Read the model definition and answer for the solid it produces. Units are mm, in the model's axes. A direction names the side the tool comes from. Coordinates: 2 decimals unless noted, no trailing zeros. Write each loop counter-clockwise with the first axis right and the second up, starting at its lowest first coordinate (ties: lowest second). Pieces come first, ordered by that corner, then holes. Notation, with made-up numbers: (-40, 67) -> (9, 67) arc R19 cw to (9, 82) -> close; hole circle Ø3 at (6.5, 74). An arc over 180 degrees is marked (long way). One line per item, written item: value. Start each with the question number.
1. For a pull along X with two mould halves and no side action, classify faces 3 (the flat face through (74, 18, 0)), 4 (the flat face through (23, 69, 337)), 5 (the cylindrical face through (90.178, 81.787, 127.677)) as pulls with the +X half, pulls with the -X half, needs draft (parallel to the pull), parting line crosses it, or undercut.
2. Find section C-C, the plane y = 85.5. State how many separate pieces and enclosed holes the cut face has, and give its area (3 significant figures).
3. Find section A-A, the plane x = 75. Write down the section's boundary in (y, z), and give its area (3 significant figures).
4. Find section D-D, the plane x = 133. Write down the section's boundary in (y, z).
5. Given P1, Ø6, axis at x = 32, y = 48, coming from the +Z side; P2, Ø8, axis at y = 78.5, z = 449, coming from the +X side; P3, Ø18, axis at x = 74, z = 113.5, coming from the +Y side, each flat-ended and moving along its own axis, determine where each tip first touches the part or whether it passes through.
6. For faces 1 (the flat face through (23, 69, 40)), 2 (the cylindrical face through (75.791, 81.787, 414.017)), determine the directions among +Z, -Z, +X, -X, +Y, -Y from which every point of the face is accessible in a straight line to the end or side of a thin tool.
7. Find section B-B, the plane z = 188. Write down the section's boundary in (x, y).
8. Consider line 1 along Y through (x, z) = (72.5, 418); line 2 along X through (y, z) = (31.5, 118); line 3 along Z through (x, y) = (77, 33). Determine where each line is inside the solid, lowest interval first.
```python
from build123d import *

# Parameters (mm, degrees)
CROQUIS1_W              = 150
CROQUIS1_H              = 102
SALIENTE_EXTRUIR1_DEPTH = 550
CORTAR_EXTRUIR1_DEPTH   = 550
CORTAR_EXTRUIR2_DEPTH   = 500
CORTAR_EXTRUIR3_DEPTH   = 3
CORTAR_EXTRUIR4_DEPTH   = 3
CROQUIS6_R              = 6.35
CORTAR_EXTRUIR5_DEPTH   = 102
CROQUIS7_R              = 18
CORTAR_EXTRUIR6_DEPTH   = 41


with BuildPart() as part:
    # Croquis1 → Saliente-Extruir1 (new body)
    with BuildSketch(Plane.XY):
        with Locations((75, 51)):
            Rectangle(CROQUIS1_W, CROQUIS1_H)
    extrude(amount=SALIENTE_EXTRUIR1_DEPTH)

    # Croquis2 → Cortar-Extruir1 (cut)
    with BuildSketch(Plane.XY.offset(550)):
        Polygon((0, 36), (46, 102), (-6.726685703, 105.184971584), align=None)
        Polygon((150, 36), (104, 102), (154.547307418, 106.586000482), align=None)
    extrude(amount=-CORTAR_EXTRUIR1_DEPTH, mode=Mode.SUBTRACT)

    # Croquis3 → Cortar-Extruir2 (cut)
    with BuildSketch(Plane.ZY):
        Polygon((0, 36), (44, 102), (0, 102), align=None)
        Polygon((550, 36), (506, 102), (550, 102), align=None)
    extrude(amount=-CORTAR_EXTRUIR2_DEPTH, mode=Mode.SUBTRACT)

    # Croquis4 → Cortar-Extruir3 (cut)
    with BuildSketch(Plane(origin=(-16.887515451, 11.770086527, 0), x_dir=(0, 0, 1), z_dir=(-0.8203981667699868, 0.5717926616881726, 0))):
        Polygon((34.193877534, 29.534334004), (78.193877534, 109.983075448), (160.193877534, 109.983075448), (116.193877534, 29.534334004), align=None)
        Polygon((193.699999945, 29.534334004), (237.699999945, 109.983075448), (319.699999945, 109.983075448), (275.699999945, 29.534334004), align=None)
        Polygon((353.206122355, 29.534334004), (397.206122355, 109.983075448), (479.206122355, 109.983075448), (435.206122355, 29.534334004), align=None)
    extrude(amount=-CORTAR_EXTRUIR3_DEPTH, mode=Mode.SUBTRACT)

    # Croquis5 → Cortar-Extruir4 (cut)
    with BuildSketch(Plane(origin=(117.845488257, 82.13473424, 0), x_dir=(0, 0, -1), z_dir=(0.8203981667699864, 0.5717926616881731, 0))):
        Polygon((-78.193877534, 24.214176195), (-34.193877534, -56.23456525), (-116.193877534, -56.23456525), (-160.193877534, 24.214176195), align=None)
        Polygon((-193.699999945, -56.23456525), (-237.699999945, 24.214176195), (-319.699999945, 24.214176195), (-275.699999945, -56.23456525), align=None)
        Polygon((-397.206122355, 24.214176195), (-353.206122355, -56.23456525), (-435.206122355, -56.23456525), (-479.206122355, 24.214176195), align=None)
    extrude(amount=-CORTAR_EXTRUIR4_DEPTH, mode=Mode.SUBTRACT)

    # Croquis6 → Cortar-Extruir5 (cut)
    with BuildSketch(Plane(origin=(0, 102, 0), x_dir=(1, 0, 0), z_dir=(0, 1, 0))):
        with Locations(Location((75, -118, 0), (0, 0, 270))):
            Circle(CROQUIS6_R)
        with Locations(Location((75, -432, 0), (0, 0, 270))):
            Circle(CROQUIS6_R)
    extrude(amount=-CORTAR_EXTRUIR5_DEPTH, mode=Mode.SUBTRACT)

    # Croquis7 → Cortar-Extruir6 (cut)
    with BuildSketch(Plane(origin=(0, 102, 0), x_dir=(1, 0, 0), z_dir=(0, 1, 0))):
        with Locations(Location((75, -118, 0), (0, 0, 270))):
            Circle(CROQUIS7_R)
        with Locations(Location((75, -432, 0), (0, 0, 270))):
            Circle(CROQUIS7_R)
    extrude(amount=-CORTAR_EXTRUIR6_DEPTH, mode=Mode.SUBTRACT)


solid = part.part
```
Answer block:
1. face 3: needs draft
1. face 4: pulls with the -X half
1. face 5: undercut
2. separate pieces: 1
2. enclosed holes: 2
2. area: 35,400 mm2
3. outline: (0, 0) -> (36, 0) -> (102, 44) -> (102, 100) -> (61, 100) -> (61, 111.65) -> (0, 111.65) -> close; (0, 124.35) -> (61, 124.35) -> (61, 136) -> (102, 136) -> (102, 414) -> (61, 414) -> (61, 425.65) -> (0, 425.65) -> close; (0, 438.35) -> (61, 438.35) -> (61, 450) -> (102, 450) -> (102, 506) -> (36, 550) -> (0, 550) -> close
3. area: 48,700 mm2
4. outline: (0, 0) -> (36, 0) -> (60.39, 16.26) -> (60.39, 50.45) -> (55.14, 48.1) -> (55.14, 130.1) -> (60.39, 132.45) -> (60.39, 209.96) -> (55.14, 207.61) -> (55.14, 289.61) -> (60.39, 291.96) -> (60.39, 369.47) -> (55.14, 367.11) -> (55.14, 449.11) -> (60.39, 451.47) -> (60.39, 533.74) -> (36, 550) -> (0, 550) -> close
5. P1: stops at z = 544
5. P2: stops at x = 119.51
5. P3: stops at y = 61
6. face 1: +Z, -Z, -X, +Y
6. face 2: +Y
7. outline: (0, 0) -> (150, 0) -> (150, 36) -> (104, 102) -> (46, 102) -> (0, 36) -> close
8. line 1: y = 0 to 61
8. line 2: x = 0 to 68.65, 81.35 to 150
8. line 3: z = 0 to 111.97, 124.03 to 425.97, 438.03 to 550
